```python
from build123d import *

# Parameters (mm, degrees)
BOSS_EXTRUDE1_DEPTH = 62.70625
CUT_EXTRUDE1_DEPTH  = 224.410663511
SKETCH3_R           = 7
SKETCH3_R_2         = 1.75
SKETCH3_R_3         = 0.5
CUT_EXTRUDE2_DEPTH  = 224.410663511


with BuildPart() as part:
    # Sketch1 → Boss-Extrude1 (new, symmetric)
    with BuildSketch(Plane.XY):
        with BuildLine():
            Line((-9.525, 149.225), (-4.7625, 149.225))
            Line((-4.7625, 149.225), (-4.7625, 0))
            ThreePointArc((-4.7625, 0), (-3.367596045, -3.367596045), (0, -4.7625))
            Line((0, -4.7625), (149.225, -4.7625))
            Line((149.225, -4.7625), (149.225, -9.525))
            Line((149.225, -9.525), (0, -9.525))
            ThreePointArc((0, -9.525), (-6.735192091, -6.735192091), (-9.525, 0))
            Line((-9.525, 0), (-9.525, 149.225))
        make_face()
    extrude(amount=BOSS_EXTRUDE1_DEPTH, both=True)

    # Sketch2 → Cut-Extrude1 (cut, through all)
    with BuildSketch(Plane(origin=(-4.7625, 0, 0), x_dir=(0, 0, -1), z_dir=(1, 0, 0))):
        with BuildLine():
            Line((-50.8, 134.9375), (-50.8, 128.5875))
            ThreePointArc((-50.8, 128.5875), (-44.45, 122.2375), (-38.1, 128.5875))
            Line((-38.1, 128.5875), (-38.1, 134.9375))
            ThreePointArc((-38.1, 134.9375), (-44.45, 141.2875), (-50.8, 134.9375))
        make_face()
        with BuildLine():
            Line((-50.8, 46.0375), (-50.8, 39.6875))
            ThreePointArc((-50.8, 39.6875), (-44.45, 33.3375), (-38.1, 39.6875))
            Line((-38.1, 39.6875), (-38.1, 46.0375))
            ThreePointArc((-38.1, 46.0375), (-44.45, 52.3875), (-50.8, 46.0375))
        make_face()
        with BuildLine():
            Line((38.1, 39.6875), (38.1, 46.0375))
            ThreePointArc((38.1, 46.0375), (44.45, 52.3875), (50.8, 46.0375))
            Line((50.8, 46.0375), (50.8, 39.6875))
            ThreePointArc((50.8, 39.6875), (44.45, 33.3375), (38.1, 39.6875))
        make_face()
        with BuildLine():
            Line((38.1, 134.9375), (38.1, 128.5875))
            ThreePointArc((38.1, 128.5875), (44.45, 122.2375), (50.8, 128.5875))
            Line((50.8, 128.5875), (50.8, 134.9375))
            ThreePointArc((50.8, 134.9375), (44.45, 141.2875), (38.1, 134.9375))
        make_face()
    cut_extrude1 = extrude(amount=-CUT_EXTRUDE1_DEPTH, mode=Mode.SUBTRACT)

    # Mirror1: Cut-Extrude1 across plane
    add(cut_extrude1.mirror(Plane(origin=(0, 0, 0), x_dir=(0, 0, 1), z_dir=(0.7071067811865475, -0.7071067811865476, 0))), mode=Mode.SUBTRACT)

    # Sketch3 → Cut-Extrude2 (cut, through all)
    with BuildSketch(Plane(origin=(-4.7625, 0, 0), x_dir=(0, 0, -1), z_dir=(1, 0, 0))):
        with Locations((-41.11625, 28.575)):
            Circle(SKETCH3_R)
        with Locations((-25.61625, 44.075)):
            Circle(SKETCH3_R_2)
        with Locations((-56.61625, 44.075)):
            Circle(SKETCH3_R_2)
        with Locations((-25.61625, 13.075)):
            Circle(SKETCH3_R_2)
        with Locations((-56.61625, 13.075)):
            Circle(SKETCH3_R_2)
        with Locations((-41.11625, 53.975)):
            Circle(SKETCH3_R_3)
    extrude(amount=-CUT_EXTRUDE2_DEPTH, mode=Mode.SUBTRACT)


solid = part.part
```
Design review of the part built by this model. Coordinates are the model's own, in mm. A direction names the side the tool comes from. Round coordinates to 2 decimals unless told otherwise and drop trailing zeros. Write each loop counter-clockwise with the first axis right and the second up, starting at its lowest first coordinate (ties: lowest second). Pieces come first, ordered by that corner, then holes.
Item 1: We need section D-D on x = 74. Write out the cut boundary in (y, z) (1 decimal), and give its area (3 significant figures).
Item 2: For faces 1 (the flat face through (-7, 43, -38.1)), 2 (the cylindrical face through (33.34, -7.11, 44.59)), list the 3-axis set-ups (+Z, -Z, +X, -X, +Y, -Y) from which the entire face can be reached by the end or side of a thin tool; tool diameter is ignored.
Item 3: Clearance check with flat-ended pins moving along their axes: pin 1 Ø22.5 at (y, z) = (28.58, 41.12) entering from -X (3 decimals); pin 2 Ø2 at (x, z) = (48.5, 31.5) entering from +Y; pin 3 Ø10 at (x, z) = (38.5, -45) entering from -Y; pin 4 Ø5 at (y, z) = (112.5, 10.5) entering from +X. State where each tip first meets the part, or that it passes through.
Item 4: For probe 1 along Y at (x, z) = (76, 24) (1 decimal); probe 2 along Y at (x, z) = (-1.5, 6.5), list the stretches that pass through material, from the lowest coordinate up.
Item 5: We need section A-A on z = -44.45. State how many separate pieces and enclosed holes the cut face has, and give its area (3 significant figures).
Item 6: The part is to be moulded in two halves that separate along Z. For faces 3 (the flat face through (-7, 132, -50.8)), 4 (the flat face through (-7, 132, 38.1)), 5 (the flat face through (35, -6, 62.706)), say which applies: +Z half, -Z half, draft (parallel to the pull), parting line (faces both ways), or undercut.
Item 7: We need section B-B on y = 25. Write out the cut boundary in (x, z) (1 decimal).
Returned:
1. outline: (-9.5, -62.7) - (-4.8, -62.7) - (-4.8, 62.7) - (-9.5, 62.7) - close
1. area: 597 mm2
2. face 1: +X, -X
2. face 2: +Y, -Y
3. pin 1: stops at x = -9.525
3. pin 2: stops at y = -4.76
3. pin 3: passes through
3. pin 4: stops at x = -4.76
4. probe 1: y = -9.5 to -4.8
4. probe 2: y = -9.41 to -4.52
5. separate pieces: 5
5. enclosed holes: 0
5. area: 1,110 mm2
6. face 3: undercut
6. face 4: undercut
6. face 5: +Z half
7. outline: (-9.5, -62.7) - (-4.8, -62.7) - (-4.8, 35.1) - (-9.5, 35.1) - close; (-9.5, 47.1) - (-4.8, 47.1) - (-4.8, 62.7) - (-9.5, 62.7) - close
